Here's how the part is built. I have some questions about the finished solid (model axes, mm). A direction names the side the tool comes from. Coordinates: 2 decimals unless noted, no trailing zeros. Loops run counter-clockwise (first coordinate to the right, second up) from the corner with the lowest first, then second, coordinate; pieces in that order, holes last.
from build123d import *

# Parameters (mm, degrees)
F4_W      = 350
F4_H      = 600
F5_DEPTH  = 600
F6_W      = 130
F6_H      = 150
F6_W_2    = 150
F6_H_2    = 130
F7_DEPTH  = 200
F8_W      = 55
F8_H      = 540
F10_DEPTH = 150


# Not quite as in the source:
# - a feature names something its author has since deleted; it is built from what else it names


with BuildPart() as f5:
    # F4 (on Top) → F5 (new body)
    with BuildSketch(Plane.XY):
        Rectangle(F4_W, F4_H)
    extrude(amount=-F5_DEPTH)

    # F6 (on face) → F7 (cut)
    with BuildSketch(Plane.XY):
        with Locations((0, -225)):
            Rectangle(F6_W, F6_H)
        with Locations((100, 0)):
            Rectangle(F6_W_2, F6_H_2)
    extrude(amount=-F7_DEPTH, mode=Mode.SUBTRACT)

    # F8 (on face) → F10 (cut)
    with BuildSketch(Plane.YZ.offset(175)):
        with Locations((123.3525127172, -270)):
            Rectangle(F8_W, F8_H)
    extrude(amount=-F10_DEPTH, mode=Mode.SUBTRACT)


solid = f5.part
Q1. Suppose I cut it at C-C on y = -29.5. Write out the boundary of the cut face in (x, z).
Q2. Please list where these lines run through material, in increasing order: probe 1 along Y at (x, z) = (103, -380); probe 2 along X at (y, z) = (-241.5, -140); probe 3 along Z at (x, y) = (107.5, 40).
Q3. For faces 5 (the flat face through (101, 150.853, -274)), 6 (the flat face through (-65, -226, -99)), 7 (the flat face through (-2, -300, -296)), which set-ups out of +Z, -Z, +X, -X, +Y, -Y let a thin tool reach every point of the face, with its end or its side?
Q4. Suppose I cut it at A-A on z = -86. Write out the boundary of the cut face in (x, y).
Q5. Suppose I cut it at D-D on x = -48.5. Write out the boundary of the cut face in (y, z).
Q6. Suppose I cut it at B-B on x = 76. Write out the boundary of the cut face in (y, z).
Q7. We'd pull the mould along Y, two halves only. Please class faces 1 (the flat face through (101, 123, -540)), 2 (the flat face through (-2, 300, -296)), 3 (the flat face through (25, -1, -99)), 4 (the flat face through (65, -226, -99)): pulls with the +Y half, pulls with the -Y half, needs draft (parallel to the pull), parting line crosses it, or undercut.
Check values:
1. outline: (-175, -600) - (175, -600) - (175, -200) - (25, -200) - (25, 0) - (-175, 0) - close
2. probe 1: y = -300 to 95.85, 150.85 to 300
2. probe 2: x = -175 to -65, 65 to 175
2. probe 3: z = -600 to -200
3. face 5: +Z, +X
3. face 6: +Z, -Y
3. face 7: +Z, -Z, +X, -X, -Y
4. outline: (-175, -300) - (-65, -300) - (-65, -150) - (65, -150) - (65, -300) - (175, -300) - (175, -65) - (25, -65) - (25, 65) - (175, 65) - (175, 95.85) - (25, 95.85) - (25, 150.85) - (175, 150.85) - (175, 300) - (-175, 300) - close
5. outline: (-300, -600) - (300, -600) - (300, 0) - (-150, 0) - (-150, -200) - (-300, -200) - close
6. outline: (-300, -600) - (300, -600) - (300, 0) - (150.85, 0) - (150.85, -540) - (95.85, -540) - (95.85, 0) - (65, 0) - (65, -200) - (-65, -200) - (-65, 0) - (-300, 0) - close
7. face 1: undercut
7. face 2: pulls with the +Y half
7. face 3: undercut
7. face 4: needs draft
